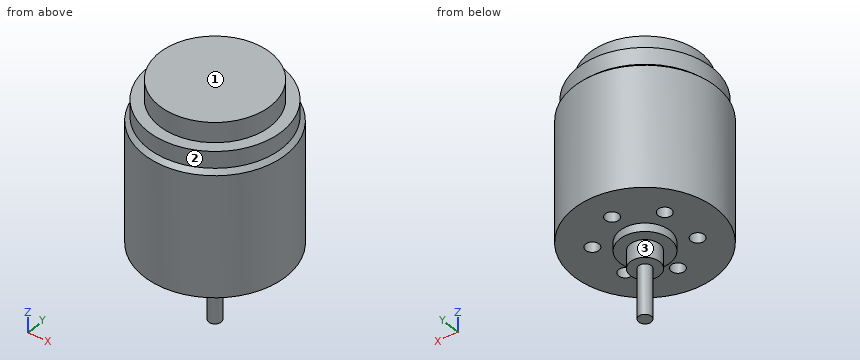
from build123d import *

# Parameters (mm, degrees)
SKETCH2_R           = 8.5
BOSS_EXTRUDE1_DEPTH = 15
CHAMFER1_SIZE       = 0.5
SKETCH3_R           = 8
BOSS_EXTRUDE2_DEPTH = 2
SKETCH4_R           = 6.65
BOSS_EXTRUDE3_DEPTH = 2.4
SKETCH5_R           = 0.8
CUT_EXTRUDE1_DEPTH  = 1.6
SKETCH6_R           = 3
BOSS_EXTRUDE4_DEPTH = 1
SKETCH7_R           = 1.75
BOSS_EXTRUDE5_DEPTH = 2.1
SKETCH8_R           = 0.75
BOSS_EXTRUDE6_DEPTH = 6


with BuildPart() as part:
    # Sketch2 → Boss-Extrude1 (new body)
    with BuildSketch(Plane.XY):
        Circle(SKETCH2_R)
    extrude(amount=BOSS_EXTRUDE1_DEPTH)

    # Chamfer1
    chamfer1_edges = [part.edges().sort_by_distance(p)[0] for p in [
        (-8.5, 0, 15),
    ]]
    chamfer(chamfer1_edges, length=CHAMFER1_SIZE)

    # Sketch3 → Boss-Extrude2 (add)
    with BuildSketch(Plane.XY.offset(15)):
        Circle(SKETCH3_R)
    extrude(amount=BOSS_EXTRUDE2_DEPTH)

    # Sketch4 → Boss-Extrude3 (add)
    with BuildSketch(Plane.XY.offset(17)):
        Circle(SKETCH4_R)
    extrude(amount=BOSS_EXTRUDE3_DEPTH)

    # Sketch5 → Cut-Extrude1 (cut)
    with BuildSketch(Plane(origin=(0, 0, 0), x_dir=(-1, 0, 0), z_dir=(0, 0, -1))):
        with Locations((0, 5)):
            Circle(SKETCH5_R)
        with Locations((4.330127019, 2.5)):
            Circle(SKETCH5_R)
        with Locations((4.330127019, -2.5)):
            Circle(SKETCH5_R)
        with Locations((0, -5)):
            Circle(SKETCH5_R)
        with Locations((-4.330127019, -2.5)):
            Circle(SKETCH5_R)
        with Locations((-4.330127019, 2.5)):
            Circle(SKETCH5_R)
    extrude(amount=-CUT_EXTRUDE1_DEPTH, mode=Mode.SUBTRACT)

    # Sketch6 → Boss-Extrude4 (add)
    with BuildSketch(Plane(origin=(0, 0, 0), x_dir=(-1, 0, 0), z_dir=(0, 0, -1))):
        Circle(SKETCH6_R)
    extrude(amount=BOSS_EXTRUDE4_DEPTH)

    # Sketch7 → Boss-Extrude5 (add)
    with BuildSketch(Plane(origin=(0, 0, -1), x_dir=(-1, 0, 0), z_dir=(0, 0, -1))):
        Circle(SKETCH7_R)
    extrude(amount=BOSS_EXTRUDE5_DEPTH)

    # Sketch8 → Boss-Extrude6 (add)
    with BuildSketch(Plane(origin=(0, 0, -3.1), x_dir=(-1, 0, 0), z_dir=(0, 0, -1))):
        Circle(SKETCH8_R)
    extrude(amount=BOSS_EXTRUDE6_DEPTH)


solid = part.part
Can you work these out from the model? Positions are in its coordinate system, mm. Face numbers are marked on the shaded views. A direction names the side the tool comes from. Give positions to 0.01 mm unless a question says otherwise; leave off trailing zeros. Write each loop counter-clockwise with the first axis right and the second up, starting at its lowest first coordinate (ties: lowest second). Pieces come first, ordered by that corner, then holes. Notation, with made-up numbers: M 37,56.25 L 60,56.25 A31 cw 60,80.25 Z; hole C -27,75.5 d1. An arc over 180 degrees is marked long. Answer in a Markdown table with one row per item. Add a question column.
Item 1: On a 3-axis mill with a long thin cutter (end or side, diameter ignored), from which of +Z, -Z, +X, -X, +Y, -Y can I reach the whole of each face in a straight line? I mean the marked faces 1, 2 and 3. Say none if no direction works.
Item 2: Please list where these lines run through material, in increasing order: L1, parallel to Y at x = 0, z = 1.1; L2, parallel to X at y = -0.25, z = 2; L3, parallel to Z at x = 0, y = -2.25.
Item 3: Imagine slicing it at C-C, the plane z = 3.75. Write out the boundary of the cut face in (x, y).
Item 4: Imagine slicing it at A-A, the plane y = 0. Write out the boundary of the cut face in (x, z), plus the area to 3 significant figures.
Item 5: For pin 1 Ø1.8 at (x, y) = (-4.5, 3) entering from -Z; pin 2 Ø1 at (y, z) = (4.5, 0.5) entering from -X; pin 3 Ø1.5 at (x, z) = (-6.5, 7) entering from +Y, each with a flat end and sliding along its axis, tell me the tip position at first contact or that it passes through.
Evaluation:
| question | item | result |
|---|---|---|
| 1 | face 1 | +Z, +X, -X, +Y, -Y |
| 1 | face 2 | +Z |
| 1 | face 3 | -Z |
| 2 | L1 | y = -8.5 to -5.8, -4.2 to 4.2, 5.8 to 8.5 |
| 2 | L2 | x = -8.5 to 8.5 |
| 2 | L3 | z = -1 to 19.4 |
| 3 | outline | C 0,0 d17 |
| 4 | outline | M -8.5,0 L -3,0 L -3,-1 L -1.75,-1 L -1.75,-3.1 L -0.75,-3.1 L -0.75,-9.1 L 0.75,-9.1 L 0.75,-3.1 L 1.75,-3.1 L 1.75,-1 L 3,-1 L 3,0 L 8.5,0 L 8.5,14.5 L 8,15 L 8,17 L 6.65,17 L 6.65,19.4 L -6.65,19.4 L -6.65,17 L -8,17 L -8,15 L -8.5,14.5 Z |
| 4 | area | 341 mm² |
| 5 | pin 1 | stops at z = 0 |
| 5 | pin 2 | stops at x = -7.5 |
| 5 | pin 3 | stops at y = 6.26 |
